The listing builds one solid part. Answer for the finished solid, in the listing's coordinates (mm). Coordinates: 2 decimals unless noted, no trailing zeros. Write each loop counter-clockwise with the first axis right and the second up, starting at its lowest first coordinate (ties: lowest second). Pieces come first, ordered by that corner, then holes.
(1) The part is cut by section C-C on y = 33. Determine the outline of the cut face in (x, z) (1 decimal).
(2) The part is cut by section B-B on z = -127. Determine the outline of the cut face in (x, y), plus the area to 3 significant figures.
(3) For a pull along Y with two mould halves and no side action, classify faces 1 (the flat face through (25, 50.8, -75)), 2 (the flat face through (0, 26, -75)), 3 (the cylindrical face through (25.76, 28.68, -137.41)), 4 (the flat face through (25, 0, -75)) as +Y half, -Y half, draft (parallel to the pull), parting line (faces both ways), or undercut.
(4) The part is cut by section D-D on z = -12.7. Determine the outline of the cut face in (x, y), plus the area to 3 significant figures.
(5) Straight lines are drawn through the part: line 1 (Z direction, x = 12.7, y = 13); line 2 (X direction, y = 38, z = -12); line 3 (Y direction, x = 21, z = -127). For each, find the intervals that lie inside material, in ascending order.
(6) The part is cut by section A-A on x = 38.1. Determine the outline of the cut face in (y, z), plus the area to 3 significant figures.
from build123d import *

# Parameters (mm, degrees)
SKETCH1_W           = 152.4
SKETCH1_H           = 50.8
BOSS_EXTRUDE1_DEPTH = 50.8
SKETCH2_R           = 10.9140625
CUT_EXTRUDE1_DEPTH  = 51.8
SKETCH3_R           = 1.5875
CUT_EXTRUDE2_DEPTH  = 51.8


with BuildPart() as part:
    # Sketch1 → Boss-Extrude1 (new body)
    with BuildSketch(Plane(origin=(0, 0, 0), x_dir=(0, 0, -1), z_dir=(1, 0, 0))):
        with Locations((76.2, 25.4)):
            Rectangle(SKETCH1_W, SKETCH1_H)
    extrude(amount=BOSS_EXTRUDE1_DEPTH)

    # Sketch2 → Cut-Extrude1 (cut, through all)
    with BuildSketch(Plane(origin=(50.8, 0, 0), x_dir=(0, 0, -1), z_dir=(1, 0, 0))):
        with Locations((127, 25.4)):
            Circle(SKETCH2_R)
    extrude(amount=-CUT_EXTRUDE1_DEPTH, mode=Mode.SUBTRACT)

    # Sketch3 → Cut-Extrude2 (cut, through all)
    with BuildSketch(Plane(origin=(0, 50.8, 0), x_dir=(1, 0, 0), z_dir=(0, 1, 0))):
        with Locations((12.7, 38.1)):
            Circle(SKETCH3_R)
        with Locations((38.1, 38.1)):
            Circle(SKETCH3_R)
        with Locations((12.7, 12.7)):
            Circle(SKETCH3_R)
        with Locations((38.1, 12.7)):
            Circle(SKETCH3_R)
    extrude(amount=-CUT_EXTRUDE2_DEPTH, mode=Mode.SUBTRACT)


solid = part.part
Model answer:
1. outline: (0, -152.4) - (50.8, -152.4) - (50.8, -134.8) - (0, -134.8) - close; (0, -119.2) - (50.8, -119.2) - (50.8, 0) - (0, 0) - close; hole circle Ø3.2 at (12.7, -38.1); hole circle Ø3.2 at (12.7, -12.7); hole circle Ø3.2 at (38.1, -38.1); hole circle Ø3.2 at (38.1, -12.7)
2. outline: (0, 0) - (50.8, 0) - (50.8, 14.49) - (0, 14.49) - close; (0, 36.31) - (50.8, 36.31) - (50.8, 50.8) - (0, 50.8) - close
2. area: 1,470 mm2
3. face 1: +Y half
3. face 2: draft
3. face 3: undercut
3. face 4: -Y half
4. outline: (0, 0) - (11.11, 0) - (11.11, 50.8) - (0, 50.8) - close; (14.29, 0) - (36.51, 0) - (36.51, 50.8) - (14.29, 50.8) - close; (39.69, 0) - (50.8, 0) - (50.8, 50.8) - (39.69, 50.8) - close
4. area: 2,260 mm2
5. line 1: z = -152.4 to -39.69, -36.51 to -14.29, -11.11 to 0
5. line 2: x = 0 to 11.28, 14.12 to 36.68, 39.52 to 50.8
5. line 3: y = 0 to 14.49, 36.31 to 50.8
6. outline: (0, -152.4) - (50.8, -152.4) - (50.8, -39.69) - (0, -39.69) - close; (0, -36.51) - (50.8, -36.51) - (50.8, -14.29) - (0, -14.29) - close; (0, -11.11) - (50.8, -11.11) - (50.8, 0) - (0, 0) - close; hole circle Ø21.83 at (25.4, -127)
6. area: 7,050 mm2
